from build123d import *

# Parameters (mm, degrees)
F0_W     = 4
F0_H     = 0.5
F1_DEPTH = 2.6
F2_R     = 1.5
F3_DEPTH = 2
F4_SIZE  = 1
F5_R     = 1
F6_R     = 1.25
F7_DEPTH = 25


with BuildPart() as f1:
    # F0 (on Right) → F1 (new body, symmetric)
    with BuildSketch(Plane.YZ):
        Polygon((0, 0), (0, 10), (3, 10), (3, 11), (0, 11), (0, 15.5), (-1.5, 15.5), (-5.5, 15.5), (-14, 15.5), (-14, 11), (-17, 11), (-17, 10), (-14, 10), (-14, 0), align=None)
        with Locations((-3.5, 15.75)):
            Rectangle(F0_W, F0_H)
    extrude(amount=F1_DEPTH, both=True)

    # F2 (on face) → F3 (join)
    with BuildSketch(Plane.XY.offset(16)):
        with Locations((0, -3.5)):
            Circle(F2_R)
    extrude(amount=F3_DEPTH)

    # F4
    f4_edges = [f1.edges().sort_by_distance(p)[0] for p in [
        (-2.6, -7, 0),
        (0, 0, 0),
        (2.6, -7, 0),
        (0, -14, 0),
    ]]
    chamfer(f4_edges, length=F4_SIZE)

    # F5
    f5_edges = [f1.edges().sort_by_distance(p)[0] for p in [
        (2.6, 0, 5.5),
        (2.6, 0, 13.25),
        (-2.6, 0, 13.25),
        (2.6, -1.5, 15.75),
        (2.6, -5.5, 15.75),
        (-2.6, -5.5, 15.75),
        (-2.6, -1.5, 15.75),
        (2.6, -14, 13.25),
        (-2.6, -14, 13.25),
        (2.6, -17, 10.5),
        (-2.6, -17, 10.5),
        (2.6, -14, 5.5),
        (-2.6, -14, 5.5),
        (2.6, 3, 10.5),
        (-2.6, 3, 10.5),
        (-2.6, 0, 5.5),
    ]]
    fillet(f5_edges, radius=F5_R)

    # F6 (on face) → F7 (cut)
    with BuildSketch(Plane.XY.offset(11)):
        with Locations((0, 2)):
            Circle(F6_R)
        with Locations((0, -16)):
            Circle(F6_R)
    extrude(amount=-F7_DEPTH, mode=Mode.SUBTRACT)


solid = f1.part
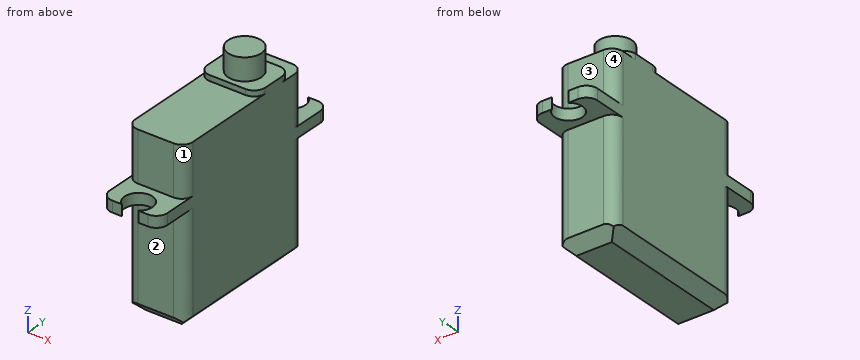
CAD build for the part. Positions are in the model's coordinates, mm. Face numbers are marked on the shaded views. A direction names the side the tool comes from. Round coordinates to 2 decimals unless told otherwise and drop trailing zeros. Order: outer loops, then holes, each group sorted by start corner. A loop starts at its lowest first (then second) coordinate and runs counter-clockwise, first axis right, second up. Notation, with made-up numbers: (23, 85.5) -> (40, 85.5) arc R18 cw to (40, 116.5) -> close; hole circle Ø2 at (86.25, 20). An arc over 180 degrees is marked (long way). Write item = value, one per line. Start each with the question number.
(1) Probe line 1 (Y direction, x = -1.05, z = 10.5); line 2 (X direction, y = -16, z = 10.65); line 3 (Z direction, x = -2, y = -14.25). List the from-to ranges inside material, lowest first. Write a range as [from, to].
(2) Pin check, flat tips, straight feed: P1, Ø3, axis at x = 0.5, y = 1, coming from the -Z side; P2, Ø3, axis at x = 0.5, y = -15, coming from the +Z side; P3, Ø1.6, axis at x = 0, z = 5.5, coming from the -Y side; P4, Ø2, axis at x = 0, y = 2, coming from the +Z side. Stop position of each tip, or through.
(3) Cut at B-B, the plane x = 0. List the corners of the cut face in (y, z).
(4) Which spindle directions (+Z, -Z, +X, -X, +Y, -Y) get a long thin tool onto all of the face, cutting with end or side? Do the marked faces 1, 2, 3 and 4. Say none if no direction does.
(5) Cut at A-A, the plane y = -3.5. List the corners of the cut face in (x, z).
(6) Cut at C-C, the plane z = 14.25. List the corners of the cut face in (x, y).
(7) Cut at D-D, the plane y = -7. List the corners of the cut face in (x, z).
Model answer:
q1.line_1 = [-17, -16.68], [-15.32, 1.32], [2.68, 3]
q1.line_2 = [-2.6, -1.25], [1.25, 2.6]
q1.line_3 = [10, 11]
q2.P1 = 0.5
q2.P2 = 15.5
q2.P3 = -14
q2.P4 = through
q3.outline = (-14.75, 10) -> (-14, 10) -> (-14, 1) -> (-13, 0) -> (-1, 0) -> (0, 1) -> (0, 10) -> (0.75, 10) -> (0.75, 11) -> (0, 11) -> (0, 15.5) -> (-1.5, 15.5) -> (-1.5, 16) -> (-2, 16) -> (-2, 18) -> (-5, 18) -> (-5, 16) -> (-5.5, 16) -> (-5.5, 15.5) -> (-14, 15.5) -> (-14, 11) -> (-14.75, 11) -> close
q4.face_1 = +Z, +X, -Y
q4.face_2 = -Z, +X, -X, -Y
q4.face_3 = +Z, +X, -X, +Y
q4.face_4 = +Z, -X, +Y
q5.outline = (-2.6, 1) -> (-1.6, 0) -> (1.6, 0) -> (2.6, 1) -> (2.6, 16) -> (1.5, 16) -> (1.5, 18) -> (-1.5, 18) -> (-1.5, 16) -> (-2.6, 16) -> close
q6.outline = (-2.6, -13) arc R1 ccw to (-1.6, -14) -> (1.6, -14) arc R1 ccw to (2.6, -13) -> (2.6, -1) arc R1 ccw to (1.6, 0) -> (-1.6, 0) arc R1 ccw to (-2.6, -1) -> close
q7.outline = (-2.6, 1) -> (-1.6, 0) -> (1.6, 0) -> (2.6, 1) -> (2.6, 15.5) -> (-2.6, 15.5) -> close
